Can you work these out from the model? Positions are in its coordinate system, mm. Face numbers are marked on the shaded views. A direction names the side the tool comes from. Give positions to 0.01 mm unless a question says otherwise; leave off trailing zeros. Loops run counter-clockwise (first coordinate to the right, second up) from the corner with the lowest first, then second, coordinate; pieces in that order, holes last. Notation, with made-up numbers: M -19.5,7.25 L 15.5,7.25 A25 cw 15.5,42.25 Z; hole C 53.5,-38 d10. An arc over 180 degrees is marked long. Answer as a JSON object with one key per item and string values.
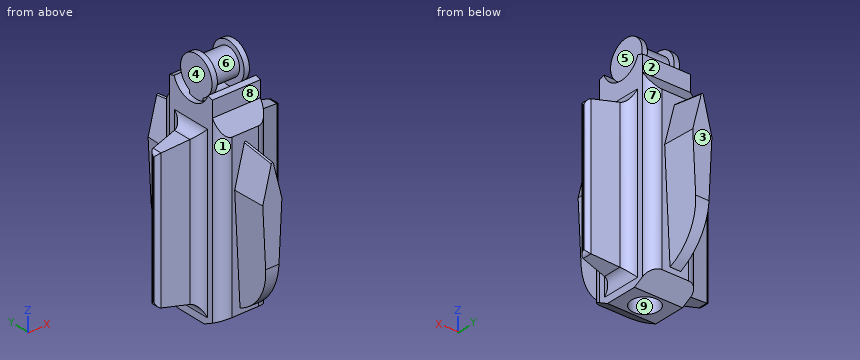
```python
from build123d import *

# Parameters (mm, degrees)
SKETCH1_R                = 3.175
BOSS_EXTRUDE1_DEPTH      = 3.175
SKETCH2_R                = 4.444999999999999
BOSS_EXTRUDE2_DEPTH      = 1.27
BOSS_EXTRUDE3_DEPTH      = 1.27
BOSS_EXTRUDE4_DEPTH      = 8.89
BOSS_EXTRUDE4_DEPTH_BACK = 2.54
SKETCH5_R                = 3.175
CUT_EXTRUDE1_DEPTH       = 12.7
FILLET1_R                = 2.54
SKETCH6_W                = 35.559999999999995
SKETCH6_H                = 5.08
BOSS_EXTRUDE5_DEPTH      = 8.889999999999999
BOSS_EXTRUDE5_TAPER      = 10.000000000000021
FILLET2_R                = 1.016
FILLET3_R                = 2.54
BOSS_EXTRUDE6_DEPTH      = 7.619999999999995
BOSS_EXTRUDE6_TAPER      = 2.000000000000002
FILLET4_R                = 0.254
FILLET5_R                = 12.7


with BuildPart() as part:
    # Sketch1 → Boss-Extrude1 (new, symmetric)
    with BuildSketch(Plane(origin=(0, 0, 0), x_dir=(0, 0, -1), z_dir=(1, 0, 0))):
        Circle(SKETCH1_R)
    extrude(amount=BOSS_EXTRUDE1_DEPTH, both=True)

    # Sketch2 → Boss-Extrude2 (add)
    with BuildSketch(Plane(origin=(3.175, 0, 0), x_dir=(0, 0, -1), z_dir=(1, 0, 0))):
        Circle(SKETCH2_R)
    boss_extrude2 = extrude(amount=BOSS_EXTRUDE2_DEPTH)

    # Mirror1: Boss-Extrude2 across plane
    add(boss_extrude2.mirror(Plane(origin=(0, 0, 0), x_dir=(0, 0, 1), z_dir=(1, 0, 0))))

    # Sketch3 → Boss-Extrude3 (add)
    with BuildSketch(Plane(origin=(4.445, 0, 0), x_dir=(0, 0, -1), z_dir=(1, 0, 0))):
        Polygon((-7.3e-16, 1.9049999999999998), (6.349999999999998, 1.9050000000000038), (6.349999999999999, -1.9049999999999998), (4.4e-16, -1.9049999999999998), align=None)
    boss_extrude3 = extrude(amount=-BOSS_EXTRUDE3_DEPTH)

    # Mirror2: Boss-Extrude3 across plane
    add(boss_extrude3.mirror(Plane(origin=(0, 0, 0), x_dir=(0, 0, 1), z_dir=(1, 0, 0))))

    # Sketch4 → Boss-Extrude4 (add, two sides: drawn at the far end of the back side and taken through both)
    with BuildSketch(Plane(origin=(-3.175, 0, 0), x_dir=(0, 0, -1), z_dir=(1, 0, 0)).offset(-BOSS_EXTRUDE4_DEPTH_BACK)):
        with BuildLine():
            Line((1.7374623280944008, 4.773638513592414), (2.1184623280943997, 6.0436385135924136))
            Line((2.1184623280943997, 6.0436385135924136), (5.928462328094399, 6.0436385135924136))
            Line((5.928462328094399, 6.0436385135924136), (9.738462328094398, 8.583638513592414))
            Line((9.738462328094398, 8.583638513592414), (47.838462328094394, 8.583638513592414))
            Line((47.838462328094394, 8.583638513592414), (50.3784623280944, 3.8099999999999996))
            Line((50.3784623280944, 3.8099999999999996), (50.3784623280944, -3.8099999999999996))
            Line((50.3784623280944, -3.8099999999999996), (47.838462328094394, -8.583638513592414))
            Line((47.838462328094394, -8.583638513592414), (9.738462328094398, -8.583638513592414))
            Line((9.738462328094398, -8.583638513592414), (5.928462328094399, -6.0436385135924136))
            Line((5.928462328094399, -6.0436385135924136), (2.1184623280943997, -6.0436385135924136))
            Line((2.1184623280943997, -6.0436385135924136), (1.7374623280944008, -4.773638513592414))
            ThreePointArc((1.7374623280944008, -4.773638513592414), (5.080000000000001, 0), (1.7374623280944008, 4.773638513592414))
        make_face()
    extrude(amount=BOSS_EXTRUDE4_DEPTH + BOSS_EXTRUDE4_DEPTH_BACK)

    # Sketch5 → Cut-Extrude1 (cut)
    with BuildSketch(Plane(origin=(0, 0, -50.3784623280944), x_dir=(-1, 0, 0), z_dir=(0, 0, -1))):
        Circle(SKETCH5_R)
    extrude(amount=-CUT_EXTRUDE1_DEPTH, mode=Mode.SUBTRACT)

    # Fillet1
    fillet1_edges = [part.edges().sort_by_distance(p)[0] for p in [
        (5.715000000000001, -8.583638513592414, -28.788462328094397),
        (-5.715, -8.583638513592414, -28.788462328094397),
        (-5.715, 8.583638513592414, -28.788462328094397),
        (5.715000000000001, 8.583638513592414, -28.788462328094397),
    ]]
    fillet(fillet1_edges, radius=FILLET1_R)

    # Sketch6 → Boss-Extrude5 (add)
    with BuildSketch(Plane(origin=(5.715000000000001, 0, 0), x_dir=(0, 0, -1), z_dir=(1, 0, 0))):
        with Locations((28.7884623280944, 0)):
            Rectangle(SKETCH6_W, SKETCH6_H)
    boss_extrude5 = extrude(amount=BOSS_EXTRUDE5_DEPTH, taper=BOSS_EXTRUDE5_TAPER)

    # Mirror3: Boss-Extrude5 across plane
    add(boss_extrude5.mirror(Plane(origin=(0, 0, 0), x_dir=(0, 0, 1), z_dir=(1, 0, 0))))

    # Fillet2
    fillet2_edges = [part.edges().sort_by_distance(p)[0] for p in [
        (14.605, -1.6e-16, -12.57600918659266),
        (14.605, -0.9724531415017433, -28.788462328094404),
        (14.605, -1.6e-16, -45.00091546959614),
        (14.605, 0.9724531415017431, -28.788462328094397),
        (-14.605, -1.6e-16, -12.57600918659266),
        (-14.605, 0.9724531415017431, -28.788462328094397),
        (-14.605, -1.6e-16, -45.00091546959614),
        (-14.605, -0.9724531415017433, -28.788462328094404),
    ]]
    fillet(fillet2_edges, radius=FILLET2_R)

    # Fillet3
    fillet3_edges = [part.edges().sort_by_distance(p)[0] for p in [
        (5.715000000000001, 0, -11.008462328094403),
        (5.715000000000001, -2.54, -28.7884623280944),
        (5.715000000000001, 0, -46.5684623280944),
        (5.715000000000001, 2.54, -28.7884623280944),
        (-5.715000000000001, 0, -11.008462328094403),
        (-5.715000000000001, -2.54, -28.7884623280944),
        (-5.715000000000001, 0, -46.5684623280944),
        (-5.715000000000001, 2.54, -28.7884623280944),
    ]]
    fillet(fillet3_edges, radius=FILLET3_R)

    # Sketch7 → Boss-Extrude6 (add)
    with BuildSketch(Plane(origin=(0, 8.583638513592414, 0), x_dir=(1, 0, 0), z_dir=(0, 1, 0))):
        Polygon((-1.27, 46.568462328094405), (-2.5399999999999983, 21.168462328094403), (0, 11.0084623280944), (2.5399999999999983, 21.168462328094403), (1.27, 46.568462328094405), align=None)
    boss_extrude6 = extrude(amount=BOSS_EXTRUDE6_DEPTH, taper=BOSS_EXTRUDE6_TAPER)

    # Mirror4: Boss-Extrude6 across plane
    add(boss_extrude6.mirror(Plane.ZX))

    # Fillet4
    fillet4_edges = [part.edges().sort_by_distance(p)[0] for p in [
        (0, 12.39363851359241, -11.557033828646649),
        (0, -12.39363851359241, -11.557033828646649),
    ]]
    fillet(fillet4_edges, radius=FILLET4_R)

    # Fillet5
    # the kernel refuses this fillet: 12.7 mm, written as the material it takes off along each edge
    with BuildSketch(Plane(origin=(29.450991141099852, -16.20363851359241, -46.30236606456729), x_dir=(0, 0.9993908270190958, -0.03489949670250097), z_dir=(-1, 0, 0))) as fillet5_piece_1:
        with BuildLine():
            CenterArc((12.295328982012144, -11.809941091943898), FILLET5_R, 111.57817847820185, 66.42182152179815)
            Line((-0.39693452113037153, -11.366717483822136), (-0.6507797911932232, -11.357853011659701))
            Line((-0.6507797911932232, -11.357853011659701), (-0.2538452700628517, 0.00886447216243529))
            Line((-0.2538452700628517, 0.00886447216243529), (-1.12e-15, 0.25399999999999656))
            ThreePointArc((-1.12e-15, 0.25399999999999656), (3.8123223637785104, 0.2539999999999965), (7.531231042467917, 0.23619882183887903))
            Line((7.531231042467917, 0.23619882183887903), (7.624644727557019, -4e-17))
        make_face()
    extrude(amount=58.90198228219971, mode=Mode.SUBTRACT)
    with BuildSketch(Plane(origin=(29.450991141099852, 16.20363851359241, -46.30236606456729), x_dir=(0, -0.9993908270190958, -0.03489949670250097), z_dir=(-1, 0, 0))) as fillet5_piece_2:
        with BuildLine():
            CenterArc((12.295328982012144, 11.809941091943898), FILLET5_R, 182, 66.42182152179817)
            Line((-0.39693452113037153, 11.366717483822136), (-0.6507797911932232, 11.357853011659701))
            Line((-0.6507797911932232, 11.357853011659701), (-0.2538452700628517, -0.00886447216243529))
            Line((-0.2538452700628517, -0.00886447216243529), (-1.12e-15, -0.25399999999999656))
            ThreePointArc((-1.12e-15, -0.25399999999999656), (3.8123223637785104, -0.2539999999999965), (7.531231042467917, -0.23619882183887903))
            Line((7.531231042467917, -0.23619882183887903), (7.624644727557019, 4e-17))
        make_face()
    extrude(amount=58.90198228219971, mode=Mode.SUBTRACT)


solid = part.part
```
1) Suppose I cut it at A-A, the plane z = 0. Write out the boundary of the cut face in (x, y) (3 decimals).
Answer list:
{"outline": "M -4.445,-4.445 L -3.175,-4.445 L -3.175,-3.175 L 3.175,-3.175 L 3.175,-4.445 L 4.445,-4.445 L 4.445,4.445 L 3.175,4.445 L 3.175,3.175 L -3.175,3.175 L -3.175,4.445 L -4.445,4.445 Z"}
2) Please list where these lines run through material, in increasing order: line 1 along X through (y, z) = (-3.5, -2.5) (3 decimals); line 2 along Y through (x, z) = (0, -43.25) (3 decimals); line 3 along Y through (x, z) = (-7.75, -41.5). Write a range as from..to.
Answer list:
{"line 1": "-4.445..-3.175, 3.175..4.445", "line 2": "-13.098..-3.175, 3.175..13.098", "line 3": "-2.18..2.18"}
3) Will these pins go through, and if not, where does the flat tip stop? pin 1 Ø6 at (x, z) = (-5.5, -26) entering from -Y; pin 2 Ø1.5 at (x, y) = (-2.5, 8) entering from +Z; pin 3 Ø1 at (x, y) = (-4, -5.5) entering from +Z.
Answer list:
{"pin 1": "y = -8.58", "pin 2": "z = -7.74", "pin 3": "z = -1.81"}
4) For the marked faces 1, 2, 3, 4 and 5, which set-ups out of +Z, -Z, +X, -X, +Y, -Y let a thin tool reach every point of the face, with its end or its side?
Answer list:
{"face 1": "+Z, -Z, -X, -Y", "face 2": "+Z, +X, -X, +Y", "face 3": "+Z, -Z, +X, -X, +Y", "face 4": "+Z, -X", "face 5": "+Z, +X"}
5) If we mould it in two halves opening along X, with no side actions, what happens to the marked faces 6, 7, 8 and 9? For each: +X half, -X half, draft (parallel to the pull), parting line (faces both ways), or undercut.
Answer list:
{"face 6": "undercut", "face 7": "+X half", "face 8": "draft", "face 9": "undercut"}
